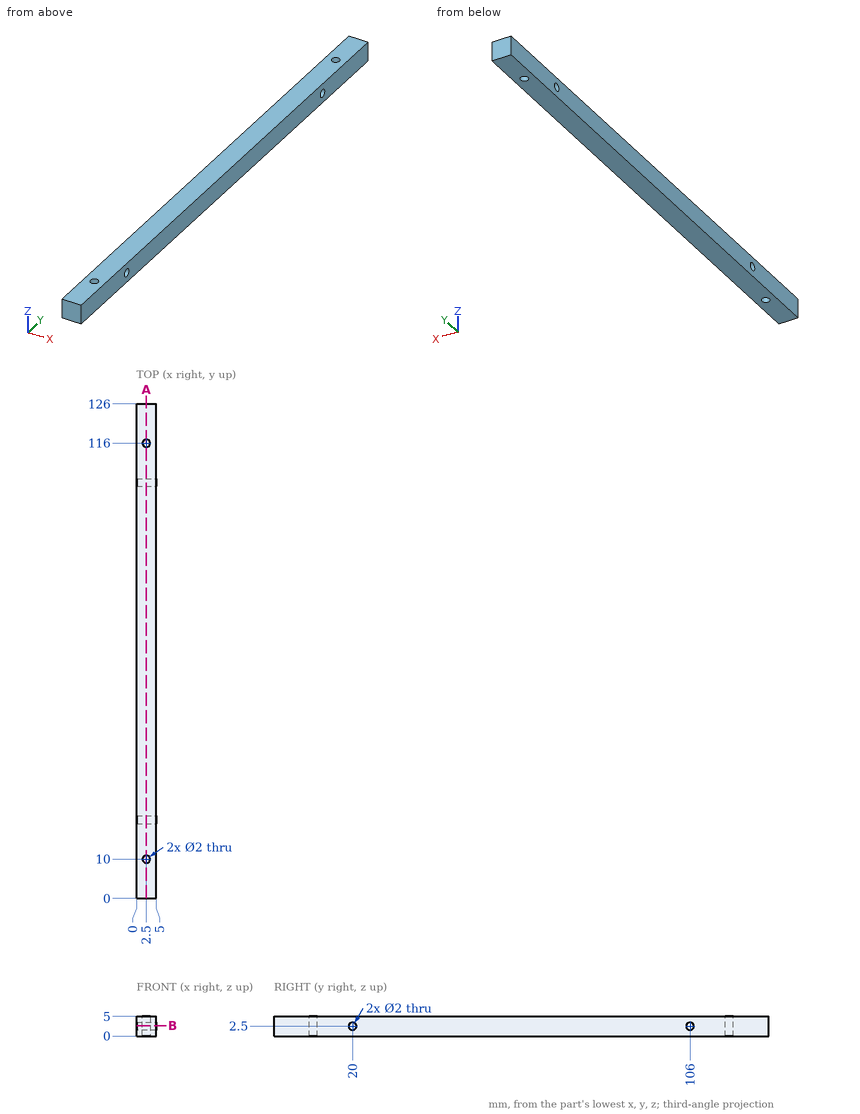
The drawing under review shows one solid part. Ordinate dimensions are in mm from its lowest x, y, z. Give positions to 0.01 mm unless a question says otherwise; leave off trailing zeros. Write each loop counter-clockwise with the first axis right and the second up, starting at its lowest first coordinate (ties: lowest second). Pieces come first, ordered by that corner, then holes. Notation, with made-up numbers: (-35.5, -12.75) -> (19.5, -12.75) arc R23 ccw to (19.5, 17.25) -> close; hole circle Ø4 at (11.25, 89). An arc over 180 degrees is marked (long way). Use CSV: the item, a comma, the result in double quotes.
Q1. Take a section at A-A, the plane x = 2.5. Write out the cut boundary in (y, z), then the cut area to 3 significant figures.
Conclusion:
outline,"(0, 0) -> (9, 0) -> (9, 5) -> (0, 5) -> close; (11, 0) -> (115, 0) -> (115, 5) -> (11, 5) -> close; (117, 0) -> (126, 0) -> (126, 5) -> (117, 5) -> close; hole circle Ø2 at (20, 2.5); hole circle Ø2 at (106, 2.5)"
area,"604 mm2"
Q2. For P1, Ø1.6, axis at y = 106, z = 2.5, coming from the -X side, flat-tipped, find the tip position at first contact; note if it passes through.
Conclusion:
P1,"through"
Q3. Take a section at B-B, the plane z = 2.65. Write out the cut boundary in (x, y).
Conclusion:
outline,"(0, 0) -> (5, 0) -> (5, 19.01) -> (0, 19.01) -> close; (0, 20.99) -> (5, 20.99) -> (5, 105.01) -> (0, 105.01) -> close; (0, 106.99) -> (5, 106.99) -> (5, 126) -> (0, 126) -> close; hole circle Ø2 at (2.5, 10); hole circle Ø2 at (2.5, 116)"
Q4. To check wall thickness, follow probe 1 along Y at (x, z) = (4.6, 2.65); probe 2 along Y at (x, z) = (2.5, 2.9); probe 3 along X at (y, z) = (116, 1.55). State the ranges of each line that lie inside material, in increasing order. Write a range as [from, to].
Conclusion:
probe 1,"[0, 19.01], [20.99, 105.01], [106.99, 126]"
probe 2,"[0, 9], [11, 19.08], [20.92, 105.08], [106.92, 115], [117, 126]"
probe 3,"[0, 1.5], [3.5, 5]"
